For this review, take the finished solid that the model builds, in its own axes (mm). A direction names the side the tool comes from. Round coordinates to 2 decimals unless told otherwise and drop trailing zeros. Write each loop counter-clockwise with the first axis right and the second up, starting at its lowest first coordinate (ties: lowest second). Pieces come first, ordered by that corner, then holes. Notation, with made-up numbers: (-25.75, 47) -> (4.25, 47) arc R31 cw to (4.25, 82) -> close; hole circle Ø2 at (-11.75, 67). An arc over 180 degrees is marked (long way). Answer in a Markdown table with one row per item.
from build123d import *

# Parameters (mm, degrees)
F2_DEPTH = 11.90625
F3_DEPTH = 11.90625


# Not quite as in the source:
# - a variable given as a bare number and used for a length is read in inches; the dataset says mm whatever the document's units were


with BuildPart() as f2:
    # F1 (on Front) → F2 (new body)
    with BuildSketch(Plane.XZ):
        with BuildLine():
            Line((914.4, 406.4), (0, 406.4))
            Line((0, 406.4), (0, 203.2))
            Line((0, 203.2), (117.3175746993, 0))
            Line((117.3175746993, 0), (222.25, 0))
            Line((222.25, 0), (222.25, 203.2))
            ThreePointArc((222.25, 203.2), (228.6, 209.55), (234.95, 203.2))
            Line((234.95, 203.2), (234.95, 0))
            Line((234.95, 0), (679.45, 0))
            Line((679.45, 0), (679.45, 203.2))
            ThreePointArc((679.45, 203.2), (685.8, 209.55), (692.15, 203.2))
            Line((692.15, 203.2), (692.15, 0))
            Line((692.15, 0), (797.0824253007, 0))
            Line((797.0824253007, 0), (914.4, 203.2))
            Line((914.4, 203.2), (914.4, 406.4))
        make_face()
        with BuildLine():
            Line((393.7, 368.3), (457.2, 368.3))
            Line((457.2, 368.3), (520.7, 368.3))
            ThreePointArc((520.7, 368.3), (539.75, 349.25), (520.7, 330.2))
            Line((520.7, 330.2), (457.2, 330.2))
            Line((457.2, 330.2), (393.7, 330.2))
            ThreePointArc((393.7, 330.2), (374.65, 349.25), (393.7, 368.3))
        make_face(mode=Mode.SUBTRACT)
    extrude(amount=F2_DEPTH)

    # F3 (add): a face of the model
    f3_faces = [f2.faces().sort_by_distance(p)[0] for p in [
        (457.2, -11.90625, 211.7591892525),
    ]]
    extrude(f3_faces, amount=F3_DEPTH)


solid = f2.part
1) Mouldability with a two-part tool opening along Z and no side actions: class faces 1 (the cylindrical face through (539.745, -11.74, 349.669)), 2 (the flat face through (679.45, -12, 100)), 3 (the flat face through (464, -12, 406.4)), 4 (the flat face through (854.92, -11.74, 100.18)) as pulls with the +Z half, pulls with the -Z half, needs draft (parallel to the pull), parting line crosses it, or undercut.
Solved:
| item | result |
|---|---|
| face 1 | undercut |
| face 2 | needs draft |
| face 3 | pulls with the +Z half |
| face 4 | pulls with the -Z half |
2) For line 1 (X direction, y = -12.25, z = 187); line 2 (X direction, y = -6, z = 144); line 3 (Z direction, x = 505, y = -8), list the stretches that pass through material, from the lowest coordinate up. Write a range as [from, to].
Solved:
| item | result |
|---|---|
| line 1 | [9.35, 222.25], [234.95, 679.45], [692.15, 905.05] |
| line 2 | [34.18, 222.25], [234.95, 679.45], [692.15, 880.22] |
| line 3 | [0, 330.2], [368.3, 406.4] |
3) Consider section D-D on x = 90. State the section outline as (y, z) points.
Solved:
| item | result |
|---|---|
| outline | (-23.81, 47.32) -> (0, 47.32) -> (0, 406.4) -> (-23.81, 406.4) -> close |
4) For faces 5 (the flat face through (458, -12, 330.2)), 6 (the flat face through (222.25, -12, 100)), 7 (the flat face through (451, 0, 206)), list the 3-axis set-ups (+Z, -Z, +X, -X, +Y, -Y) from which the entire face can be reached by the end or side of a thin tool; tool diameter is ignored.
Solved:
| item | result |
|---|---|
| face 5 | +Y, -Y |
| face 6 | -Z, +Y, -Y |
| face 7 | +Z, -Z, +X, -X, +Y |
5) Consider section B-B on z = 94. State the section outline as (x, y) points.
Solved:
| item | result |
|---|---|
| outline | (63.05, -23.81) -> (222.25, -23.81) -> (222.25, 0) -> (63.05, 0) -> close; (234.95, -23.81) -> (679.45, -23.81) -> (679.45, 0) -> (234.95, 0) -> close; (692.15, -23.81) -> (851.35, -23.81) -> (851.35, 0) -> (692.15, 0) -> close |
6) Consider section C-C on x = 850.5. State the section outline as (y, z) points, then the cut area to 3 significant figures.
Solved:
| item | result |
|---|---|
| outline | (-23.81, 92.52) -> (0, 92.52) -> (0, 406.4) -> (-23.81, 406.4) -> close |
| area | 7,470 mm² |
7) Consider section A-A on y = -5.5. State the section outline as (x, z) points.
Solved:
| item | result |
|---|---|
| outline | (0, 203.2) -> (117.32, 0) -> (222.25, 0) -> (222.25, 203.2) arc R6.35 cw to (234.95, 203.2) -> (234.95, 0) -> (679.45, 0) -> (679.45, 203.2) arc R6.35 cw to (692.15, 203.2) -> (692.15, 0) -> (797.08, 0) -> (914.4, 203.2) -> (914.4, 406.4) -> (0, 406.4) -> close; hole (393.7, 330.2) -> (520.7, 330.2) arc R19.05 ccw to (520.7, 368.3) -> (393.7, 368.3) arc R19.05 ccw to start |
8) Clearance check with flat-ended pins moving along their axes: pin 1 Ø10 at (x, z) = (414.5, 303.5) entering from +Y; pin 2 Ø12 at (y, z) = (-10.5, 115.5) entering from -X; pin 3 Ø1.5 at (y, z) = (-13, 49.5) entering from -X; pin 4 Ø6 at (y, z) = (-19, 139.5) entering from -X. State where each tip first meets the part, or that it passes through.
Solved:
| item | result |
|---|---|
| pin 1 | y = 0 |
| pin 2 | x = 47.17 |
| pin 3 | x = 88.31 |
| pin 4 | x = 35.05 |
